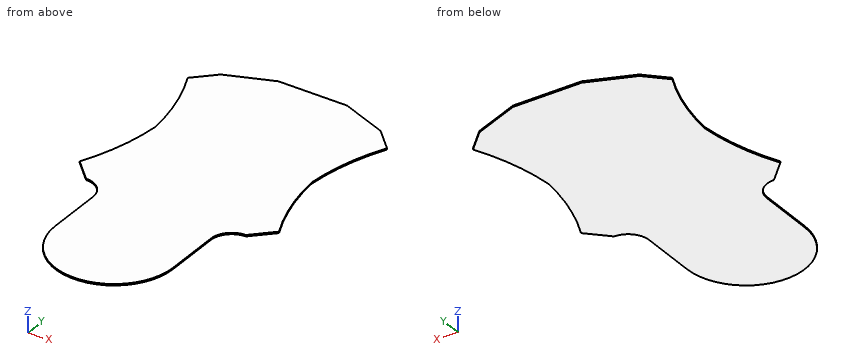
```python
from build123d import *

# Parameters (mm, degrees)
BOSS_EXTRUDE1_DEPTH = 2


with BuildPart() as part:
    # Sketch1 → Boss-Extrude1 (new body)
    with BuildSketch(Plane.XY):
        with BuildLine():
            Line((-142.766074481, 114.481803233), (-114.481803233, 142.766074481))
            Line((-114.481803233, 142.766074481), (-49.267584828, 168.204347178))
            Line((-49.267584828, 168.204347178), (49.267584828, 168.204347178))
            Line((49.267584828, 168.204347178), (114.481803233, 142.766074481))
            Line((114.481803233, 142.766074481), (142.766074481, 114.481803233))
            ThreePointArc((142.766074481, 114.481803233), (122.165206788, 58.660093881), (112.192625845, 0))
            ThreePointArc((112.192625845, 0), (122.165206788, -58.660093881), (142.766074481, -114.481803233))
            Line((142.766074481, -114.481803233), (114.481803233, -142.766074481))
            ThreePointArc((114.481803233, -142.766074481), (93.268599798, -151.552871045), (84.481803233, -172.766074481))
            Line((84.481803233, -172.766074481), (84.481803233, -252.766074481))
            ThreePointArc((84.481803233, -252.766074481), (0, -337.247877714), (-84.481803233, -252.766074481))
            Line((-84.481803233, -252.766074481), (-84.481803233, -172.766074481))
            ThreePointArc((-84.481803233, -172.766074481), (-93.268599798, -151.552871045), (-114.481803233, -142.766074481))
            Line((-114.481803233, -142.766074481), (-142.766074481, -114.481803233))
            ThreePointArc((-142.766074481, -114.481803233), (-122.165206788, -58.660093881), (-112.192625845, 0))
            ThreePointArc((-112.192625845, 0), (-122.165206788, 58.660093881), (-142.766074481, 114.481803233))
        make_face()
    extrude(amount=BOSS_EXTRUDE1_DEPTH)


solid = part.part
```
For this review, take the finished solid that the model builds, in its own axes (mm). Coordinates: 2 decimals unless noted, no trailing zeros. Loops run counter-clockwise (first coordinate to the right, second up) from the corner with the lowest first, then second, coordinate; pieces in that order, holes last.
1. For line 1 (X direction, y = 1, z = 0.5); line 2 (X direction, y = -208.5, z = 1.85); line 3 (Y direction, x = -35, z = 1.95), list the stretches that pass through material, from the lowest coordinate up.
2. Add section A-A, the plane z = 0.65. Give the boundary of the cut face in (x, y).
3. Insertion check: P1, Ø8, axis at x = -37, y = -132, coming from the -Z side. The pin has a flat end and moves straight along its axis. Give the tip position at first contact, or say it passes through.
4. Add section B-B, the plane x = -58.5. Give the boundary of the cut face in (y, z).
5. Add section C-C, the plane y = 9.5. Give the boundary of the cut face in (x, z), then the cut area to 3 significant figures.
Result:
1. line 1: x = -112.27 to 112.27
1. line 2: x = -84.48 to 84.48
1. line 3: y = -329.66 to 168.2
2. outline: (-142.77, -114.48) - (-114.48, -142.77) arc R30 cw to (-84.48, -172.77) - (-84.48, -252.77) arc R84.48 ccw to (84.48, -252.77) - (84.48, -172.77) arc R30 cw to (114.48, -142.77) - (142.77, -114.48) arc R321.84 cw to (112.19, 0) arc R321.84 cw to (142.77, 114.48) - (114.48, 142.77) - (49.27, 168.2) - (-49.27, 168.2) - (-114.48, 142.77) - (-142.77, 114.48) arc R321.84 cw to (-112.19, 0) arc R321.84 cw to start
3. P1: stops at z = 0
4. outline: (-313.72, 0) - (164.6, 0) - (164.6, 2) - (-313.72, 2) - close
5. outline: (-113.06, 0) - (113.06, 0) - (113.06, 2) - (-113.06, 2) - close
5. area: 452 mm2
